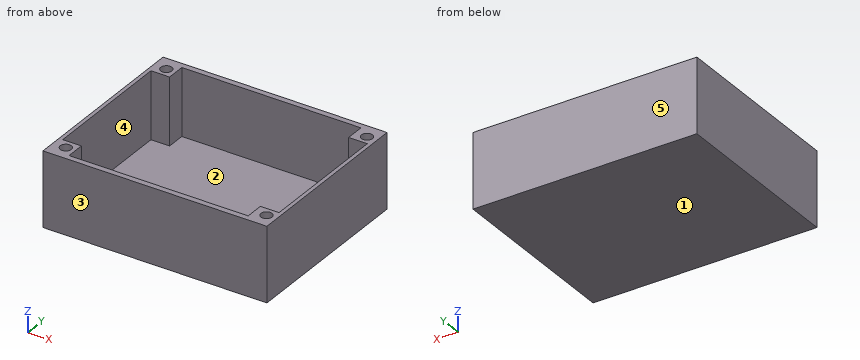
```python
from build123d import *

# Parameters (mm, degrees)
F0_W     = 60
F0_H     = 49
F1_DEPTH = 20
F2_W     = 58
F2_H     = 46
F3_DEPTH = 18
F4_W     = 5
F4_H     = 5
F5_DEPTH = 18
F6_R     = 1.5
F7_DEPTH = 10


with BuildPart() as f1:
    # F0 (on Top) → F1 (new body)
    with BuildSketch(Plane.XY):
        Rectangle(F0_W, F0_H)
    extrude(amount=F1_DEPTH)

    # F2 (on face) → F3 (cut)
    with BuildSketch(Plane.XY.offset(20)):
        Rectangle(F2_W, F2_H)
    extrude(amount=-F3_DEPTH, mode=Mode.SUBTRACT)

    # F4 (on face) → F5 (join)
    with BuildSketch(Plane.XY.offset(2)):
        with Locations((-26.5, -20.5)):
            Rectangle(F4_W, F4_H)
        with Locations((26.5, -20.5)):
            Rectangle(F4_W, F4_H)
        with Locations((-26.5, 20.5)):
            Rectangle(F4_W, F4_H)
        with Locations((26.5, 20.5)):
            Rectangle(F4_W, F4_H)
    extrude(amount=F5_DEPTH)

    # F6 (on face) → F7 (cut)
    with BuildSketch(Plane.XY.offset(20)):
        with Locations((-26.5, -20.5)):
            Circle(F6_R)
        with Locations((-26.5, 20.5)):
            Circle(F6_R)
        with Locations((27.266302, 20.5)):
            Circle(F6_R)
        with Locations((27.266302, -20.5)):
            Circle(F6_R)
    extrude(amount=-F7_DEPTH, mode=Mode.SUBTRACT)


solid = f1.part
```
The model under review builds one solid part; all positions refer to its coordinate system, in mm. Face numbers are marked on the shaded views. A direction names the side the tool comes from. Coordinates: 2 decimals unless noted, no trailing zeros. Write each loop counter-clockwise with the first axis right and the second up, starting at its lowest first coordinate (ties: lowest second). Pieces come first, ordered by that corner, then holes. Notation, with made-up numbers: (-19.5, 2.25) - (18.5, 2.25) arc R26 ccw to (18.5, 32.25) - close; hole circle Ø9 at (-14.5, 74). An arc over 180 degrees is marked (long way). Answer in a Markdown table with one row per item. Add a question column.
Q1. To check wall thickness, follow line 1 along Y through (x, z) = (-26.5, 14.25); line 2 along Y through (x, z) = (-5.5, 17.5); line 3 along X through (y, z) = (-18.5, 13.75). State the ranges of each line that lie inside material, in increasing order. Write a range as from..to.
Q2. Consider section C-C on z = 17.25. Give the boundary of the cut face in (x, y).
Q3. Draft analysis for pull direction Y (two halves, no side actions). For the marked faces 3, 4 and 5, state which applies: +Y half, -Y half, draft (parallel to the pull), parting line (faces both ways), or undercut.
Q4. For the marked faces 1 and 2, list the 3-axis set-ups (+Z, -Z, +X, -X, +Y, -Y) from which the entire face can be reached by the end or side of a thin tool; tool diameter is ignored.
Q5. Consider section A-A on x = -26.5. Give the boundary of the cut face in (y, z).
Q6. Clearance check with flat-ended pins moving along their axes: pin 1 (12 mm diameter, centred on x = 3.5, y = -8.5, fed in from -Z); pin 2 (0.9 mm diameter, centred on x = -26, y = 20.5, fed in from +Z); pin 3 (23 mm diameter, centred on x = 1, y = -7.5, fed in from +Z). State where each tip first meets the part, or that it passes through.
Q7. Consider section B-B on y = -20.5. Give the boundary of the cut face in (x, z).
Q8. Consider section D-D on y = 8. Give the boundary of the cut face in (x, z), then the cut area to 3 significant figures.
Answers below:
| question | item | result |
|---|---|---|
| 1 | line 1 | -24.5..-22, -19..-18, 18..19, 22..24.5 |
| 1 | line 2 | -24.5..-23, 23..24.5 |
| 1 | line 3 | -30..-24, 24..30 |
| 2 | outline | (-30, -24.5) - (30, -24.5) - (30, 24.5) - (-30, 24.5) - close; hole (-29, -18) - (-24, -18) - (-24, -23) - (24, -23) - (24, -18) - (29, -18) - (29, 18) - (24, 18) - (24, 23) - (-24, 23) - (-24, 18) - (-29, 18) - close; hole circle Ø3 at (-26.5, -20.5); hole circle Ø3 at (-26.5, 20.5); hole circle Ø3 at (27.27, -20.5); hole circle Ø3 at (27.27, 20.5) |
| 3 | face 3 | -Y half |
| 3 | face 4 | undercut |
| 3 | face 5 | +Y half |
| 4 | face 1 | -Z, +X, -X, +Y, -Y |
| 4 | face 2 | +Z |
| 5 | outline | (-24.5, 0) - (24.5, 0) - (24.5, 20) - (22, 20) - (22, 10) - (19, 10) - (19, 20) - (18, 20) - (18, 2) - (-18, 2) - (-18, 20) - (-19, 20) - (-19, 10) - (-22, 10) - (-22, 20) - (-24.5, 20) - close |
| 6 | pin 1 | z = 0 |
| 6 | pin 2 | z = 10 |
| 6 | pin 3 | z = 2 |
| 7 | outline | (-30, 0) - (30, 0) - (30, 20) - (28.77, 20) - (28.77, 10) - (25.77, 10) - (25.77, 20) - (24, 20) - (24, 2) - (-24, 2) - (-24, 20) - (-25, 20) - (-25, 10) - (-28, 10) - (-28, 20) - (-30, 20) - close |
| 8 | outline | (-30, 0) - (30, 0) - (30, 20) - (29, 20) - (29, 2) - (-29, 2) - (-29, 20) - (-30, 20) - close |
| 8 | area | 156 mm² |
